from build123d import *

# Parameters (mm, degrees)
SKETCH1_R           = 2.125
BOSS_EXTRUDE1_DEPTH = 5
SKETCH2_R           = 2
CUT_EXTRUDE1_DEPTH  = 10
SKETCH5_R           = 6.5
BOSS_EXTRUDE2_DEPTH = 15.5
BOSS_EXTRUDE3_DEPTH = 8
SKETCH8_R           = 2
CUT_EXTRUDE2_DEPTH  = 34.5


with BuildPart() as part:
    # Sketch1 → Boss-Extrude1 (new body)
    with BuildSketch(Plane(origin=(0, 0, 0), x_dir=(1, 0, 0), z_dir=(0, 1, 0))):
        with BuildLine():
            Line((-7, 79), (-12.469480556, 0.872957419))
            ThreePointArc((-12.469480556, 0.872957419), (-12.499997094, -0.008523482), (-12.468278459, -0.889961946))
            Line((-12.468278459, -0.889961946), (-7, -77.5))
            ThreePointArc((-7, -77.5), (0, -84.5), (7, -77.5))
            Line((7, -77.5), (12.468278459, -0.889961946))
            ThreePointArc((12.468278459, -0.889961946), (12.499997094, -0.008523482), (12.469480556, 0.872957419))
            Line((12.469480556, 0.872957419), (7, 79))
            ThreePointArc((7, 79), (0, 86), (-7, 79))
        make_face()
        Circle(SKETCH1_R, mode=Mode.SUBTRACT)
    boss_extrude1 = extrude(amount=BOSS_EXTRUDE1_DEPTH)

    # Sketch2 → Cut-Extrude1 (cut)
    with BuildSketch(Plane(origin=(0, 5, 0), x_dir=(1, 0, 0), z_dir=(0, 1, 0))):
        with Locations((0, 79)):
            Circle(SKETCH2_R)
        with Locations((0, -79)):
            Circle(SKETCH2_R)
    cut_extrude1 = extrude(amount=-CUT_EXTRUDE1_DEPTH, mode=Mode.SUBTRACT)

    # Sketch5 → Boss-Extrude2 (add)
    with BuildSketch(Plane.XZ):
        Circle(SKETCH5_R)
    extrude(amount=BOSS_EXTRUDE2_DEPTH)

    # Sketch6 → Boss-Extrude3 (add)
    with BuildSketch(Plane(origin=(0, 5, 0), x_dir=(1, 0, 0), z_dir=(0, 1, 0))):
        with BuildLine():
            Line((-9.4069118, 44.619239575), (9.4069118, 44.619239575))
            Line((9.4069118, 44.619239575), (12.469480556, 0.872957419))
            ThreePointArc((12.469480556, 0.872957419), (12.499997094, -0.008523482), (12.468278459, -0.889961946))
            Line((12.468278459, -0.889961946), (9.346965992, -44.619239575))
            Line((9.346965992, -44.619239575), (-9.346965992, -44.619239575))
            Line((-9.346965992, -44.619239575), (-12.468278459, -0.889961946))
            ThreePointArc((-12.468278459, -0.889961946), (-12.499997094, -0.008523482), (-12.469480556, 0.872957419))
            Line((-12.469480556, 0.872957419), (-9.4069118, 44.619239575))
        make_face()
    extrude(amount=BOSS_EXTRUDE3_DEPTH)

    # Mirror1: Boss-Extrude1, Cut-Extrude1 across plane
    add(boss_extrude1.mirror(Plane.ZX.offset(9)))
    add(cut_extrude1.mirror(Plane.ZX.offset(9)), mode=Mode.SUBTRACT)

    # Sketch8 → Cut-Extrude2 (cut, through all)
    with BuildSketch(Plane.XZ.offset(15.5)):
        Circle(SKETCH8_R)
    extrude(amount=-CUT_EXTRUDE2_DEPTH, mode=Mode.SUBTRACT)


solid = part.part
Here's how the part is built. I have some questions about the finished solid (model axes, mm). A direction names the side the tool comes from. Coordinates: 2 decimals unless noted, no trailing zeros. Write each loop counter-clockwise with the first axis right and the second up, starting at its lowest first coordinate (ties: lowest second). Pieces come first, ordered by that corner, then holes.
Item 1: If I drill on line 1 (Z direction, x = 0, y = 1.45) (3 decimals); line 2 (Y direction, x = -0.5, z = 72); line 3 (Z direction, x = -0.25, y = -8), over which ranges is the centre line in solid material (lowest first)?
Item 2: I want a section at B-B on z = 79. Write out the boundary of the cut face in (x, y).
Item 3: I want a section at A-A on z = -68. Write out the boundary of the cut face in (x, y).
Item 4: Will these pins go through, and if not, where does the flat tip stop? pin 1 (4.5 mm diameter, centred on x = 0, z = 0.5, fed in from +Y); pin 2 (3 mm diameter, centred on x = -7.5, z = -59, fed in from -Y); pin 3 (10 mm diameter, centred on y = -1, z = 13.5, fed in from +X); pin 4 (2.5 mm diameter, centred on x = 0, z = 0, fed in from +Y).
Item 5: On a 3-axis mill with a long thin cutter (end or side, diameter ignored), from which of +Z, -Z, +X, -X, +Y, -Y can I reach the whole of each face in a straight line? I mean faces 1 (the flat face through (0, 9, 44.619)), 2 (the cylindrical face through (1.142, 15.535, -1.792)), 3 (the flat face through (0, 5, -61)), 4 (the cylindrical face through (-5.158, -7.642, -3.955)). Say none if no direction works.
Item 6: If we mould it in two halves opening along Z, with no side actions, what happens to faces 5 (the cylindrical face through (1.142, 2.465, -1.792)), 6 (the flat face through (3, 18, -2)), 7 (the cylindrical face through (0, 16, -86))? For each: +Z half, -Z half, draft (parallel to the pull), parting line (faces both ways), or undercut.
Item 7: I want a section at D-D on x = 0. Count the separate pieces of the cut face and the enclosed holes in it, and give its area (3 significant figures).
Item 8: I want a section at C-C on y = -12. Write out the boundary of the cut face in (x, z), and give its area (3 significant figures).
Findings below:
1. line 1: z = -86 to -81, -77 to -2.125, 2.125 to 77, 81 to 84.5
1. line 2: y = 0 to 5, 13 to 18
1. line 3: z = -6.5 to -1.98, 1.98 to 6.5
2. outline: (-6.84, 0) - (-2, 0) - (-2, 5) - (-6.84, 5) - close; (-6.84, 13) - (-2, 13) - (-2, 18) - (-6.84, 18) - close; (2, 0) - (6.84, 0) - (6.84, 5) - (2, 5) - close; (2, 13) - (6.84, 13) - (6.84, 18) - (2, 18) - close
3. outline: (-7.77, 0) - (7.77, 0) - (7.77, 5) - (-7.77, 5) - close; (-7.77, 13) - (7.77, 13) - (7.77, 18) - (-7.77, 18) - close
4. pin 1: stops at y = 18
4. pin 2: stops at y = 0
4. pin 3: stops at x = 11.92
4. pin 4: passes through
5. face 1: +Z, +X, -X
5. face 2: +Y
5. face 3: -Z, +X, -X
5. face 4: -Y
6. face 5: undercut
6. face 6: draft
6. face 7: -Z half
7. separate pieces: 6
7. enclosed holes: 0
7. area: 2,400 mm2
8. outline: circle Ø13 at (0, 0); hole circle Ø4 at (0, 0)
8. area: 120 mm2
